```python
from build123d import *

# Parameters (mm, degrees)
SKETCH_1_W          = 40
SKETCH_1_H          = 10
EXTRUDE_1_DEPTH     = 6
CUT_EXTRUDE_1_REACH = 23.471
SKETCH_2_R          = 1.6
FILLET_1_R          = 3


with BuildPart() as part:
    # 草图1 → 凸台-拉伸1 (new body)
    with BuildSketch(Plane(origin=(0, 0, 0), x_dir=(1, 0, 0), z_dir=(0, 1, 0))):
        Rectangle(SKETCH_1_W, SKETCH_1_H)
    extrude(amount=EXTRUDE_1_DEPTH)

    # 草图2 → 切除-拉伸1 (cut, up to next)
    with BuildSketch(Plane(origin=(0, 6, 0), x_dir=(1, 0, 0), z_dir=(0, 1, 0)), mode=Mode.PRIVATE) as cut_extrude_1_sk1:
        with Locations(Location((-15.612495, 0, 0), (0, 0, 270))):
            Circle(SKETCH_2_R)
    cut_extrude_1_tool1 = extrude(cut_extrude_1_sk1.sketch, amount=-CUT_EXTRUDE_1_REACH, mode=Mode.PRIVATE) & part.part
    # 草图2 → 切除-拉伸1 (cut, up to next)
    with BuildSketch(Plane(origin=(0, 6, 0), x_dir=(1, 0, 0), z_dir=(0, 1, 0)), mode=Mode.PRIVATE) as cut_extrude_1_sk2:
        with Locations(Location((15.612495, 0, 0), (0, 0, 270))):
            Circle(SKETCH_2_R)
    cut_extrude_1_tool2 = extrude(cut_extrude_1_sk2.sketch, amount=-CUT_EXTRUDE_1_REACH, mode=Mode.PRIVATE) & part.part
    add(cut_extrude_1_tool1.solids().sort_by_distance((-15.612495, 6, 0))[0], mode=Mode.SUBTRACT)
    add(cut_extrude_1_tool2.solids().sort_by_distance((15.612495, 6, 0))[0], mode=Mode.SUBTRACT)

    # 圆角1
    fillet_1_edges = [part.edges().sort_by_distance(p)[0] for p in [
        (20, 3, 5),
        (-20, 3, 5),
        (-20, 3, -5),
        (20, 3, -5),
    ]]
    fillet(fillet_1_edges, radius=FILLET_1_R)


solid = part.part
```
Geometry check sheet. Reference: the model listing, model coordinates, mm. Give positions to 0.01 mm unless a question says otherwise; leave off trailing zeros. Write each loop counter-clockwise with the first axis right and the second up, starting at its lowest first coordinate (ties: lowest second). Pieces come first, ordered by that corner, then holes.
1) Section check A-A, the plane z = 0. Record the boundary of the cut face in (x, y), and give its area (3 significant figures).
2) Material ranges on L1, parallel to X at y = 3.4, z = 0; L2, parallel to X at y = 1.05, z = 0.5; L3, parallel to Z at x = -17, y = 3.9, recorded low to high.
3) Gauge pin test, flat ends, axial feed: pin 1 (1.9 mm diameter, centred on x = -15.61, z = 0, fed in from +Y); pin 2 (5 mm diameter, centred on x = 15.61, z = 0, fed in from -Y). Record the tip position at first contact, or that the pin passes through.
4) Section check B-B, the plane y = 4.4. Record the boundary of the cut face in (x, z), and give its area (3 significant figures).
5) Section check C-C, the plane z = 3.5. Record the boundary of the cut face in (x, y).
6) Release check for a two-part mould opening along Z. For faces 1 (the cylindrical face through (17.2, 3, -0.2)), 2 (the flat face through (20, 3, 0)), 3 (the cylindrical face through (-19.14, 3.04, 4.1)) record: pulls with the +Z half, pulls with the -Z half, needs draft (parallel to the pull), parting line crosses it, or undercut.
Computed:
1. outline: (-20, 0) - (-17.21, 0) - (-17.21, 6) - (-20, 6) - close; (-14.01, 0) - (14.01, 0) - (14.01, 6) - (-14.01, 6) - close; (17.21, 0) - (20, 0) - (20, 6) - (17.21, 6) - close
1. area: 202 mm2
2. L1: x = -20 to -17.21, -14.01 to 14.01, 17.21 to 20
2. L2: x = -20 to -17.13, -14.09 to 14.09, 17.13 to 20
2. L3: z = -5 to -0.8, 0.8 to 5
3. pin 1: passes through
3. pin 2: stops at y = 0
4. outline: (-20, -2) arc R3 ccw to (-17, -5) - (17, -5) arc R3 ccw to (20, -2) - (20, 2) arc R3 ccw to (17, 5) - (-17, 5) arc R3 ccw to (-20, 2) - close; hole circle Ø3.2 at (-15.61, 0); hole circle Ø3.2 at (15.61, 0)
4. area: 376 mm2
5. outline: (-19.6, 0) - (19.6, 0) - (19.6, 6) - (-19.6, 6) - close
6. face 1: undercut
6. face 2: needs draft
6. face 3: pulls with the +Z half
